```python
from build123d import *

# Parameters (mm, degrees)
BOSS_EXTRUDE1_DEPTH = 4
BOSS_EXTRUDE2_DEPTH = 80
SKETCH3_R           = 8.5
CUT_EXTRUDE1_DEPTH  = 171
SKETCH4_W           = 68
SKETCH4_H           = 18.002499925
CUT_EXTRUDE2_DEPTH  = 116
SKETCH5_W           = 23
SKETCH5_H           = 47
CUT_EXTRUDE3_DEPTH  = 110.266506281
SKETCH8_W           = 47
SKETCH8_H           = 37.321718457
CUT_EXTRUDE6_DEPTH  = 3.266506281
FILLET2_R           = 5
FILLET3_R           = 5
FILLET4_R           = 5
SKETCH9_W           = 106
SKETCH9_H           = 50.845410363
CUT_EXTRUDE7_DEPTH  = 92
FILLET16_R          = 10
FILLET18_R          = 3
CUT_EXTRUDE9_DEPTH  = 90


with BuildPart() as part:
    # Sketch1 → Boss-Extrude1 (new body)
    with BuildSketch(Plane(origin=(0, 0, 0), x_dir=(1, 0, 0), z_dir=(0, 1, 0))):
        Polygon((0, 152), (0, 101.37), (75, 101.37), (75, 191.351980657), (75, 192.37), (0, 192.37), align=None)
    extrude(amount=BOSS_EXTRUDE1_DEPTH)

    # Sketch2 → Boss-Extrude2 (add)
    with BuildSketch(Plane(origin=(0, 0, 0), x_dir=(-1, 0, 0), z_dir=(0, -1, 0))):
        Polygon((26, 91.37), (26, 176.99818396), (26, 195.45), (-80, 195.45), (-80, 176.99818396), (-80, 91.37), align=None)
        Polygon((-75, 192), (-75, 192.37), (0, 192.37), (0, 101.37), (-75, 101.37), align=None, mode=Mode.SUBTRACT)
    extrude(amount=-BOSS_EXTRUDE2_DEPTH)

    # Sketch3 → Cut-Extrude1 (cut)
    with BuildSketch(Plane.XY.offset(18)):
        with Locations((34.765402097, 21.5)):
            Circle(SKETCH3_R)
    extrude(amount=-CUT_EXTRUDE1_DEPTH, mode=Mode.SUBTRACT)

    # Sketch4 → Cut-Extrude2 (cut)
    with BuildSketch(Plane(origin=(0, 4, 0), x_dir=(1, 0, 0), z_dir=(0, 1, 0))):
        with Locations((34.5, 183.368750038)):
            Rectangle(SKETCH4_W, SKETCH4_H)
    extrude(amount=-CUT_EXTRUDE2_DEPTH, mode=Mode.SUBTRACT)

    # Sketch5 → Cut-Extrude3 (cut)
    with BuildSketch(Plane(origin=(0, 80, 0), x_dir=(1, 0, 0), z_dir=(0, 1, 0))):
        with Locations((-13, 166.95)):
            Rectangle(SKETCH5_W, SKETCH5_H)
    extrude(amount=-CUT_EXTRUDE3_DEPTH, mode=Mode.SUBTRACT)

    # Sketch8 → Cut-Extrude6 (cut)
    with BuildSketch(Plane.ZY.offset(1.5)):
        with Locations((-166.95181604, 33.429515658)):
            Rectangle(SKETCH8_W, SKETCH8_H)
    extrude(amount=-CUT_EXTRUDE6_DEPTH, mode=Mode.SUBTRACT)

    # Fillet2
    # the kernel refuses this fillet: 5 mm, written as the material it takes off along each edge
    with BuildSketch(Plane(origin=(-21, 75, -190.45), x_dir=(0, 0, -1), z_dir=(0, 1, 0))) as fillet2_piece_1_section:
        Polygon((0, 0), (FILLET2_R, 0), (FILLET2_R, FILLET2_R), (0, FILLET2_R), align=None)
    fillet2_piece_1 = extrude(amount=FILLET2_R, mode=Mode.PRIVATE)
    fillet2_piece_1 = fillet2_piece_1 - Plane(origin=(-21, 75, -190.45), x_dir=(0.7071067811865475, 0, 0.7071067811865475), z_dir=(0, 1, 0)) * Sphere(FILLET2_R, mode=Mode.PRIVATE)
    add(fillet2_piece_1, mode=Mode.SUBTRACT)
    with BuildSketch(Plane(origin=(80, -12.5, -91.37), x_dir=(-1, 0, 0), z_dir=(0, 1, 0))) as fillet2_piece_2:
        with BuildLine():
            CenterArc((FILLET2_R, -FILLET2_R), FILLET2_R, 90, 90)
            Line((0, -FILLET2_R), (0, 0))
            Line((0, 0), (FILLET2_R, 0))
        make_face()
    extrude(amount=105, mode=Mode.SUBTRACT)
    with BuildSketch(Plane(origin=(92.5, 80, -91.37), x_dir=(0, 0, -1), z_dir=(-1, 0, 0))) as fillet2_piece_3:
        with BuildLine():
            CenterArc((FILLET2_R, FILLET2_R), FILLET2_R, 180, 90)
            Line((0, FILLET2_R), (0, 0))
            Line((0, 0), (FILLET2_R, 0))
        make_face()
    extrude(amount=131, mode=Mode.SUBTRACT)
    with BuildSketch(Plane(origin=(-26, -12.5, -195.45), x_dir=(0, 0, 1), z_dir=(0, 1, 0))) as fillet2_piece_4:
        with BuildLine():
            CenterArc((FILLET2_R, FILLET2_R), FILLET2_R, 180, 90)
            Line((0, FILLET2_R), (0, 0))
            Line((0, 0), (FILLET2_R, 0))
        make_face()
    extrude(amount=87.5, mode=Mode.SUBTRACT)
    with BuildSketch(Plane(origin=(-26, 80, -78.87), x_dir=(1, 0, 0), z_dir=(0, 0, -1))) as fillet2_piece_5:
        with BuildLine():
            CenterArc((FILLET2_R, FILLET2_R), FILLET2_R, 180, 90)
            Line((0, FILLET2_R), (0, 0))
            Line((0, 0), (FILLET2_R, 0))
        make_face()
    extrude(amount=111.58, mode=Mode.SUBTRACT)
    with BuildSketch(Plane(origin=(80, -12.5, -195.45), x_dir=(-1, 0, 0), z_dir=(0, 1, 0))) as fillet2_piece_6:
        with BuildLine():
            CenterArc((FILLET2_R, FILLET2_R), FILLET2_R, 180, 90)
            Line((0, FILLET2_R), (0, 0))
            Line((0, 0), (FILLET2_R, 0))
        make_face()
    extrude(amount=105, mode=Mode.SUBTRACT)
    with BuildSketch(Plane(origin=(-21, 80, -195.45), x_dir=(0, 0, 1), z_dir=(1, 0, 0))) as fillet2_piece_7:
        with BuildLine():
            CenterArc((FILLET2_R, FILLET2_R), FILLET2_R, 180, 90)
            Line((0, FILLET2_R), (0, 0))
            Line((0, 0), (FILLET2_R, 0))
        make_face()
    extrude(amount=113.5, mode=Mode.SUBTRACT)

    # Fillet3
    # the kernel refuses this fillet: 5 mm, written as the material it takes off along each edge
    with BuildSketch(Plane(origin=(-21, 75, -96.37), x_dir=(0, 0, 1), z_dir=(-1, 0, 0))) as fillet3_piece_1_section:
        Polygon((0, 0), (FILLET3_R, 0), (FILLET3_R, FILLET3_R), (0, FILLET3_R), align=None)
    fillet3_piece_1 = extrude(amount=FILLET3_R, mode=Mode.PRIVATE)
    fillet3_piece_1 = fillet3_piece_1 - Plane(origin=(-21, 75, -96.37), x_dir=(0, -0.7071067811865475, -0.7071067811865475), z_dir=(-1, 0, 0)) * Sphere(FILLET3_R, mode=Mode.PRIVATE)
    add(fillet3_piece_1, mode=Mode.SUBTRACT)
    with BuildSketch(Plane(origin=(-26, -12.5, -91.37), x_dir=(0, 0, -1), z_dir=(0, 1, 0))) as fillet3_piece_2:
        with BuildLine():
            CenterArc((FILLET3_R, -FILLET3_R), FILLET3_R, 90, 90)
            Line((0, -FILLET3_R), (0, 0))
            Line((0, 0), (FILLET3_R, 0))
        make_face()
    extrude(amount=87.5, mode=Mode.SUBTRACT)

    # Fillet4
    # the kernel refuses this fillet: 5 mm, written as the material it takes off along each edge
    with BuildSketch(Plane(origin=(75, 75, -190.45), x_dir=(1, 0, 0), z_dir=(0, 1, 0))) as fillet4_piece_1_section:
        Polygon((0, 0), (FILLET4_R, 0), (FILLET4_R, FILLET4_R), (0, FILLET4_R), align=None)
    fillet4_piece_1 = extrude(amount=FILLET4_R, mode=Mode.PRIVATE)
    fillet4_piece_1 = fillet4_piece_1 - Plane(origin=(75, 75, -190.45), x_dir=(-0.7071067811865475, 0, 0.7071067811865475), z_dir=(0, 1, 0)) * Sphere(FILLET4_R, mode=Mode.PRIVATE)
    add(fillet4_piece_1, mode=Mode.SUBTRACT)
    with BuildSketch(Plane(origin=(75, 75, -96.37), x_dir=(1, 0, 0), z_dir=(0, 1, 0))) as fillet4_piece_2_section:
        Polygon((0, 0), (FILLET4_R, 0), (FILLET4_R, -FILLET4_R), (0, -FILLET4_R), align=None)
    fillet4_piece_2 = extrude(amount=FILLET4_R, mode=Mode.PRIVATE)
    fillet4_piece_2 = fillet4_piece_2 - Plane(origin=(75, 75, -96.37), x_dir=(-0.7071067811865475, 0, -0.7071067811865475), z_dir=(0, 1, 0)) * Sphere(FILLET4_R, mode=Mode.PRIVATE)
    add(fillet4_piece_2, mode=Mode.SUBTRACT)
    with BuildSketch(Plane(origin=(80, 80, -190.45), x_dir=(-1, 0, 0), z_dir=(0, 0, 1))) as fillet4_piece_3:
        with BuildLine():
            CenterArc((FILLET4_R, FILLET4_R), FILLET4_R, 180, 90)
            Line((0, FILLET4_R), (0, 0))
            Line((0, 0), (FILLET4_R, 0))
        make_face()
    extrude(amount=94.08, mode=Mode.SUBTRACT)

    # Sketch9 → Cut-Extrude7 (cut)
    with BuildSketch(Plane(origin=(0, 80, 0), x_dir=(1, 0, 0), z_dir=(0, 1, 0))):
        with Locations((27, 116.792705182)):
            Rectangle(SKETCH9_W, SKETCH9_H)
    extrude(amount=-CUT_EXTRUDE7_DEPTH, mode=Mode.SUBTRACT)

    # Fillet16
    # the kernel refuses this fillet: 10 mm, written as the material it takes off along each edge
    with BuildSketch(Plane(origin=(75, 101.650635095, -142.215410363), x_dir=(0, 0, -1), z_dir=(0, -1, 0))) as fillet16_piece_1:
        with BuildLine():
            CenterArc((8.660254038, 10), FILLET16_R, 210, 60)
            Line((0, 5), (0, 0))
            Line((0, 0), (8.660254038, 0))
        make_face()
    extrude(amount=97.650635095, mode=Mode.SUBTRACT)

    # Fillet18
    # the kernel refuses this fillet: 3 mm, written as the material it takes off along each edge
    with BuildSketch(Plane(origin=(0, 4, -142.215410363), x_dir=(-1, 0, 0), z_dir=(0, 1, 0))) as fillet18_piece_1:
        with BuildLine():
            CenterArc((FILLET18_R, -FILLET18_R), FILLET18_R, 90, 90)
            Line((0, -FILLET18_R), (0, 0))
            Line((0, 0), (FILLET18_R, 0))
        make_face()
    extrude(amount=83.5, mode=Mode.SUBTRACT)

    # Sketch10 → Cut-Extrude9 (cut)
    with BuildSketch(Plane.XZ):
        Polygon((80, -190.45), (80, -142.215410363), (0, -142.215410363), (0, -195.45), (80, -195.45), align=None)
    extrude(amount=-CUT_EXTRUDE9_DEPTH, mode=Mode.SUBTRACT)


solid = part.part
```
Geometry check sheet. Reference: the model listing, model coordinates, mm. A direction names the side the tool comes from. Give positions to 0.01 mm unless a question says otherwise; leave off trailing zeros. Write each loop counter-clockwise with the first axis right and the second up, starting at its lowest first coordinate (ties: lowest second). Pieces come first, ordered by that corner, then holes. Notation, with made-up numbers: (-6, -5.75) -> (29, -5.75) arc R16 ccw to (29, 5.25) -> close; hole circle Ø6 at (59, -36). An arc over 180 degrees is marked (long way). Use one line per item in the form item = value.
Item 1: Mould release check, pull along X, two halves, no side actions. Record for faces 1 (the flat face through (-1.5, 58, -167)), 2 (the cylindrical face through (-25.554, 77.063, -165.995)), 3 (the flat face through (-0.7, 4, -142.8)): released by +X, released by -X, zero draft, split by the parting line, or undercut.
Results list:
face_1 = undercut
face_2 = released by -X
face_3 = zero draft
Item 2: Sectioned sample at A-A on z = -150. Enter the section's corners in (x, y).
Results list:
outline = (-26, 0) -> (-24.5, 0) -> (-24.5, 78.57) arc R5 ccw to (-26, 75) -> close; (-1.5, 0) -> (0, 0) -> (0, 14.77) -> (-1.5, 14.77) -> close; (-1.5, 52.09) -> (0, 52.09) -> (0, 80) -> (-1.5, 80) -> close
Item 3: Access from +Z, -Z, +X, -X, +Y, -Y to the whole of each face (thin tool, end or side, straight path). Record for faces 4 (the flat face through (-1, 52.09, -167)), 5 (the flat face through (-13, 41, -143.45)), 6 (the flat face through (-1, 0, -175)), 7 (the cylindrical face through (-1.306, 41.468, -142.739)), 8 (the flat face through (-11, 37, -195.45)).
Results list:
face_4 = +X
face_5 = +Y, -Y
face_6 = +Z, -Z, +X, -X, -Y
face_7 = +Z, +X, +Y
face_8 = -Z, +X, -X, +Y, -Y
Item 4: Sectioned sample at C-C on y = 71. Enter the section's corners in (x, z).
Results list:
outline = (-26, -190.45) arc R5 ccw to (-21, -195.45) -> (0, -195.45) -> (0, -145.22) arc R3 ccw to (-3, -142.22) -> (-26, -142.22) -> close; hole (-24.5, -190.45) -> (-1.5, -190.45) -> (-1.5, -143.45) -> (-24.5, -143.45) -> close
Item 5: Depth check by flat-ended pin: pin 1 Ø12 at (y, z) = (40.5, -180.5) entering from +X; pin 2 Ø0.8 at (x, y) = (-1, 31.5) entering from +Z. Enter the tip coordinate at first touch or a pass-through.
Results list:
pin_1 = -24.5
pin_2 = -142.68
Item 6: Sectioned sample at B-B on x = -19.5. Enter the section's corners in (y, z), plus the area to 3 significant figures.
Results list:
outline = (0, -195.45) -> (75, -195.45) arc R5 ccw to (80, -190.45) -> (0, -190.45) -> close; (0, -143.45) -> (80, -143.45) -> (80, -142.22) -> (0, -142.22) -> close
area = 493 mm2
Item 7: Scan lines: line 1 (X direction, y = 6.5, z = -181.5); line 2 (Z direction, x = -20, y = 27). Record each from-to range of solid material in increasing order.
Results list:
line_1 = -26 to -24.5, -1.5 to 0
line_2 = -195.45 to -190.45, -143.45 to -142.22
